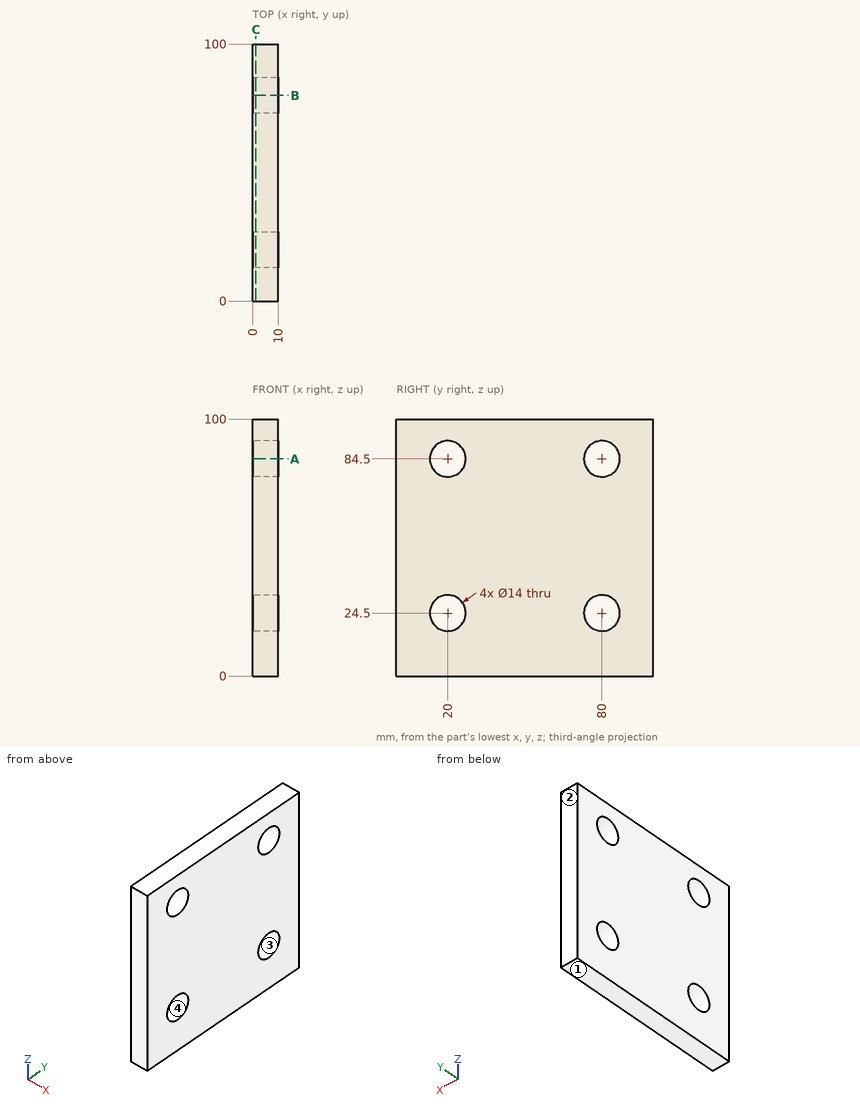
Input: dimensioned drawing with shaded views. Units: mm. Origin: part minimum x, y, z. Coordinates: 2 decimals unless noted, no trailing zeros. Write each loop counter-clockwise with the first axis right and the second up, starting at its lowest first coordinate (ties: lowest second). Pieces come first, ordered by that corner, then holes. Notation, with made-up numbers: M 67,-27 L 71,-27 A15 ccw 71,-8 Z; hole C 59,33.5 d8. An arc over 180 degrees is marked long. Answer as a JSON object with one key per item and string values. Group by question number.
(1) Section C-C on x = 1.25. Output: boundary loops of the cut face in (y, z).
(2) Contact query for a flat-ended pin moving along its axis: P1, Ø12.5, axis at y = 80, z = 84.5, coming from the +X side. Output: stop coordinate, or through.
(3) Mould query, pull axis Y, two halves, no side actions, for the marked faces 1, 2, 3 and 4. Classes: pulls with the +Y half, pulls with the -Y half, needs draft (parallel to the pull), parting line crosses it, or undercut.
(4) Section B-B on y = 80. Output: boundary loops of the cut face in (x, z).
(5) Section A-A on z = 84.5. Output: boundary loops of the cut face in (x, y), plus the area to 3 significant figures.
(6) Ray query, line 1 along Z through (x, y) = (8.25, 20); line 2 along Y through (x, z) = (3.5, 24); line 3 along Z through (x, y) = (3.75, 83). Return the intervals inside material, ascending. Write a range as [from, to].
Result set:
{
 "1": {"outline": "M 0,0 L 100,0 L 100,100 L 0,100 Z; hole C 20,24.5 d14; hole C 20,84.5 d14; hole C 80,24.5 d14; hole C 80,84.5 d14"},
 "2": {"P1": "passes through"},
 "3": {"face 1": "needs draft", "face 2": "pulls with the +Y half", "face 3": "undercut", "face 4": "undercut"},
 "4": {"outline": "M 0,0 L 10,0 L 10,17.5 L 0,17.5 Z; M 0,31.5 L 10,31.5 L 10,77.5 L 0,77.5 Z; M 0,91.5 L 10,91.5 L 10,100 L 0,100 Z"},
 "5": {"outline": "M 0,0 L 10,0 L 10,13 L 0,13 Z; M 0,27 L 10,27 L 10,73 L 0,73 Z; M 0,87 L 10,87 L 10,100 L 0,100 Z", "area": "720 mm2"},
 "6": {"line 1": "z = [0, 17.5], [31.5, 77.5], [91.5, 100]", "line 2": "y = [0, 13.02], [26.98, 73.02], [86.98, 100]", "line 3": "z = [0, 18.18], [30.82, 78.18], [90.82, 100]"}
}
